Read the model definition and answer for the solid it produces. Units are mm, in the model's axes. Face numbers are marked on the shaded views. A direction names the side the tool comes from. Coordinates: 2 decimals unless noted, no trailing zeros. Order: outer loops, then holes, each group sorted by start corner. A loop starts at its lowest first (then second) coordinate and runs counter-clockwise, first axis right, second up. Notation, with made-up numbers: (20.5, -33) -> (48.5, -33) arc R21 cw to (48.5, -15) -> close; hole circle Ø7 at (59.5, -30). An arc over 180 degrees is marked (long way). Answer in a Markdown table with one row per item.
Autodesk Inventor part; units mm, degrees
ref_plane "YZ Plane" through (0, 0, 0) normal (1, 0, 0) x (0, 1, 0)
ref_plane "XZ Plane" through (0, 0, 0) normal (0, 1, 0) x (-1, 0, 0)
ref_plane "XY Plane" through (0, 0, 0) normal (0, 0, 1) x (1, 0, 0)
sketch "Sketch1" plane through (0, 0, 0) normal (0, 0, 1) x (1, 0, 0)
  line L0 (0, 0) -> (26, 0)
  line L1 (26, 0) -> (26, 3)
  line L2 (22, 7) -> (4, 7)
  line L3 (0, 3) -> (0, 0)
  arc A0 (4, 7) -> (0, 3) centre (4, 3) ccw
  arc A1 (26, 3) -> (22, 7) centre (22, 3) ccw
  line L4 (4, 10.5) -> (22, 10.5)
  arc A2 (29.5, 3) -> (22, 10.5) centre (22, 3) ccw
  line L5 (29.5, 3) -> (29.5, -3.5)
  line L6 (29.5, -3.5) -> (-3.5, -3.5)
  line L7 (-3.5, -3.5) -> (-3.5, 3)
  arc A3 (4, 10.5) -> (-3.5, 3) centre (4, 3) ccw
  line L8 (0, 0) -> (0, -3.5)
  line L9 (26, 0) -> (26, -3.5)
  line L10 (-3.5, -3.5) -> (-17.5, -3.5)
  line L11 (-17.5, -3.5) -> (-17.5, 1.5)
  line L12 (-17.5, 1.5) -> (-3.5, 1.5)
  line L13 (-3.5, 1.5) -> (-3.5, -3.5)
  line L14 (29.5, -3.5) -> (43.5, -3.5)
  line L15 (43.5, -3.5) -> (43.5, 1.5)
  line L16 (43.5, 1.5) -> (29.5, 1.5)
  line L17 (29.5, 1.5) -> (29.5, -3.5)
  point P0 (26, 7)
  point P1 (0, 7)
  dimension "d0" = 26
  dimension "d1" = 7
  dimension "d2" = 4
  dimension "d3" = 3.5
  dimension "d6" = 14
  dimension "d7" = 5
  dimension "d8" = 14
  dimension "d9" = 5
extrude "Extrusion2" add sketch "Sketch1" along normal blind 20 contours L8 L6 L7 A3 L4 A2 L5 L9 L1 A1 L2 A0 L3 | L10 L11 L12 L7 | L5 L16 L15 L14
fillet "Fillet1" radius 7 2 edges at (29.5, 1.5, 10) (-3.5, 1.5, 10)
fillet "Fillet3" radius 6 4 edges at (-17.5, -1, 20) (-17.5, -1, 0) (43.5, -1, 20) (43.5, -1, 0)
sketch "Sketch2" plane through (35.4164, 1.5, 20) normal (0, 1, 0) x (1, 0, 0)
  circle A0 centre (1.0836, 10) radius 2.75
  line L0 (8.0836, 14) -> (8.0836, 6)
  circle A1 centre (1.0836, 10) radius 5.5
  line L1 (-13.4164, 20) -> (-31.4164, 20)
  line L2 (-22.4164, 20) -> (-22.4164, 23.3018)
  circle A2 centre (-45.9164, 10) radius 2.75
  circle A3 centre (-45.9164, 10) radius 5.5
  point P0 (-35.4164, 20)
  point P1 (8.0836, 10)
  dimension "d16" = 7
  dimension "d17" = 5.5
  dimension "d18" = 11
extrude "Extrusion3" cut sketch "Sketch2" against normal through all contours A0 | A2
extrude "Extrusion4" cut sketch "Sketch2" along normal through all contours A0 | A1 | A2 | A3
properties part number "large-cable-clip"
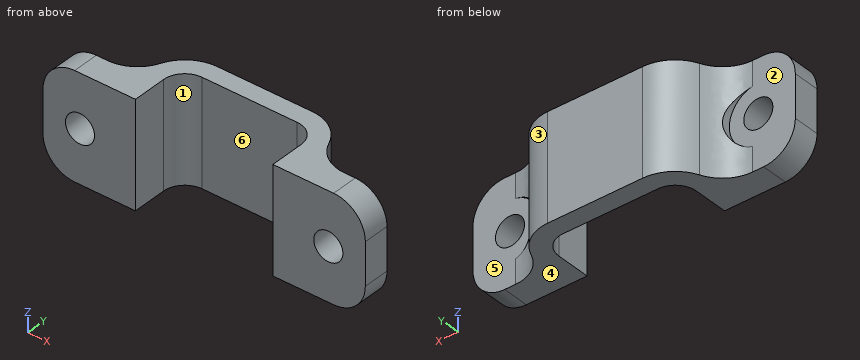
Q1. The part is cut by section A-A (x = 36.5). Write down the section's boundary in (y, z).
Outcome:
| item | result |
|---|---|
| outline | (-3.5, 0) -> (1.5, 0) -> (1.5, 7.25) -> (-3.5, 7.25) -> close; (-3.5, 12.75) -> (1.5, 12.75) -> (1.5, 20) -> (-3.5, 20) -> close |
Q2. Consider line 1 (X direction, y = 0.35, z = 10); line 2 (Z direction, x = -10.5, y = -2.45); line 3 (Y direction, x = 16.5, z = 17.25). Determine where each line is inside the solid, lowest interval first.
Outcome:
| item | result |
|---|---|
| line 1 | -17.5 to -13.25, -7.75 to 0, 26 to 33.75, 39.25 to 43.5 |
| line 2 | 0 to 7.25, 12.75 to 20 |
| line 3 | 7 to 10.5 |
Q3. Given pin 1 (2 mm diameter, centred on x = 19, z = 7, fed in from -Y); pin 2 (2 mm diameter, centred on y = 9, z = 7.5, fed in from +X); pin 3 (6.5 mm diameter, centred on x = 40, z = 14, fed in from +Y); pin 4 (4.5 mm diameter, centred on x = -10.5, z = 10, fed in from -Y), each flat-ended and moving along its own axis, determine where each tip first touches the part or whether it passes through.
Outcome:
| item | result |
|---|---|
| pin 1 | y = 7 |
| pin 2 | x = 27.59 |
| pin 3 | y = 1.5 |
| pin 4 | through |
Q4. The part is cut by section D-D (x = 10). Write down the section's boundary in (y, z).
Outcome:
| item | result |
|---|---|
| outline | (7, 0) -> (10.5, 0) -> (10.5, 20) -> (7, 20) -> close |
Q5. For a pull along Z with two mould halves and no side action, classify the marked faces 4, 5 and 6 as pulls with the +Z half, pulls with the -Z half, needs draft (parallel to the pull), parting line crosses it, or undercut.
Outcome:
| item | result |
|---|---|
| face 4 | pulls with the -Z half |
| face 5 | undercut |
| face 6 | needs draft |
Q6. For the marked faces 1, 2 and 3, determine the directions among +Z, -Z, +X, -X, +Y, -Y from which every point of the face is accessible in a straight line to the end or side of a thin tool.
Outcome:
| item | result |
|---|---|
| face 1 | +Z, -Z, -Y |
| face 2 | -X, +Y |
| face 3 | +Z, -Z, +X, +Y |
Q7. The part is cut by section B-B (z = 10). Give the number of separate pieces and of enclosed holes in the cut face, then the cut area to 3 significant figures.
Outcome:
| item | result |
|---|---|
| separate pieces | 3 |
| enclosed holes | 0 |
| area | 264 mm² |
Q8. The part is cut by section C-C (x = -10). Write down the section's boundary in (y, z).
Outcome:
| item | result |
|---|---|
| outline | (-3.5, 0) -> (1.5, 0) -> (1.5, 7.3) -> (-3.5, 7.3) -> close; (-3.5, 12.7) -> (1.5, 12.7) -> (1.5, 20) -> (-3.5, 20) -> close |
